from build123d import *

# Parameters (mm, degrees)
CHAMFER1_SIZE = 0.1


with BuildPart() as part:
    # Sketch1 → Revolve1 (revolve)
    with BuildSketch(Plane(origin=(0, 0, 0), x_dir=(0, 0, -1), z_dir=(1, 0, 0)), mode=Mode.PRIVATE) as revolve1_sk:
        Polygon((-2, 2), (-2, -2), (-2.5, -2), (-2.5, -1.5), (-2.6, -1.5), (-2.6, -1.9), (-3.35, -1.9), (-3.75, -1.5), (-4, -1.5), (-4, -2), (-4.5, -2), (-4.5, 2), (-4, 2), (-4, 1.5), (-3.75, 1.5), (-3.35, 1.9), (-2.6, 1.9), (-2.6, 1.5), (-2.5, 1.5), (-2.5, 2), align=None)
    revolve(revolve1_sk.sketch.rotate(Axis((0, -2, 0), (0, 1, 0)), 180), axis=Axis((0, -2, 0), (0, 1, 0)))

    # Chamfer1
    chamfer1_edges = [part.edges().sort_by_distance(p)[0] for p in [
        (0, 2, 4.5),
        (0, -2, 4.5),
        (0, -2, 2),
        (0, 2, 2),
    ]]
    chamfer(chamfer1_edges, length=CHAMFER1_SIZE)


solid = part.part
Part model, mm, in its own coordinate system. A direction names the side the tool comes from. Give positions to 0.01 mm unless a question says otherwise; leave off trailing zeros. Order: outer loops, then holes, each group sorted by start corner. A loop starts at its lowest first (then second) coordinate and runs counter-clockwise, first axis right, second up. Notation, with made-up numbers: (51.5, -1) -> (108.5, -1) arc R23 cw to (108.5, 21) -> close; hole circle Ø11 at (-6.5, 44). An arc over 180 degrees is marked (long way). Use one line per item in the form item = value.
(1) Drill centre lines: line 1 (Y direction, x = 3.25, z = -2.25); line 2 (X direction, y = 0.7, z = -1.5); line 3 (X direction, y = 1.05, z = 1.75). Where is each one in solid material? Low to high. Write a range as from..to.
Solution:
line_1 = -1.5..1.5
line_2 = -4.24..-1.32, 1.32..4.24
line_3 = -4.15..-0.97, 0.97..4.15
(2) Saw through at B-B (y = 0.2). Write the cut outline in (x, z), then the cut area to 3 significant figures.
Solution:
outline = circle Ø9 at (0, 0); hole circle Ø4 at (0, 0)
area = 51.1 mm²
(3) Saw through at A-A (y = 1.75). Write the cut outline in (x, z), then the cut area to 3 significant figures.
Solution:
outline = circle Ø9 at (0, 0); circle Ø7 at (0, 0); circle Ø5 at (0, 0); hole circle Ø8 at (0, 0); hole circle Ø5.2 at (0, 0); hole circle Ø4 at (0, 0)
area = 37.7 mm²
(4) Tool access for faces 1 (the face through (2, 1.9, -2)), 2 (the face through (2, 0, 0)), 3 (the face through (2, -1.9, 2)): list every direction of +Z, -Z, +X, -X, +Y, -Y with a clear straight run to the whole face (end or side of a thin tool).
Solution:
face_1 = +Y
face_2 = +Y, -Y
face_3 = -Y
(5) Flat gauge pins, fed straight in: P1, Ø1, axis at x = 1.5, y = 0.5, coming from the +Z side; P2, Ø1.5, axis at x = 1, y = -0.5, coming from the -Z side. Where does each tip first touch, or does it go through?
Solution:
P1 = 4.39
P2 = -4.49
